Geometry check sheet. Reference: drawing and pictorial views, mm from the part's lowest x, y, z. Coordinates: 2 decimals unless noted, no trailing zeros. Write each loop counter-clockwise with the first axis right and the second up, starting at its lowest first coordinate (ties: lowest second). Pieces come first, ordered by that corner, then holes. Notation, with made-up numbers: (-14.5, 67.5) -> (14.5, 67.5) arc R20 ccw to (14.5, 81.5) -> close; hole circle Ø2 at (54.25, 17). An arc over 180 degrees is marked (long way). Use a Markdown table: item, result.
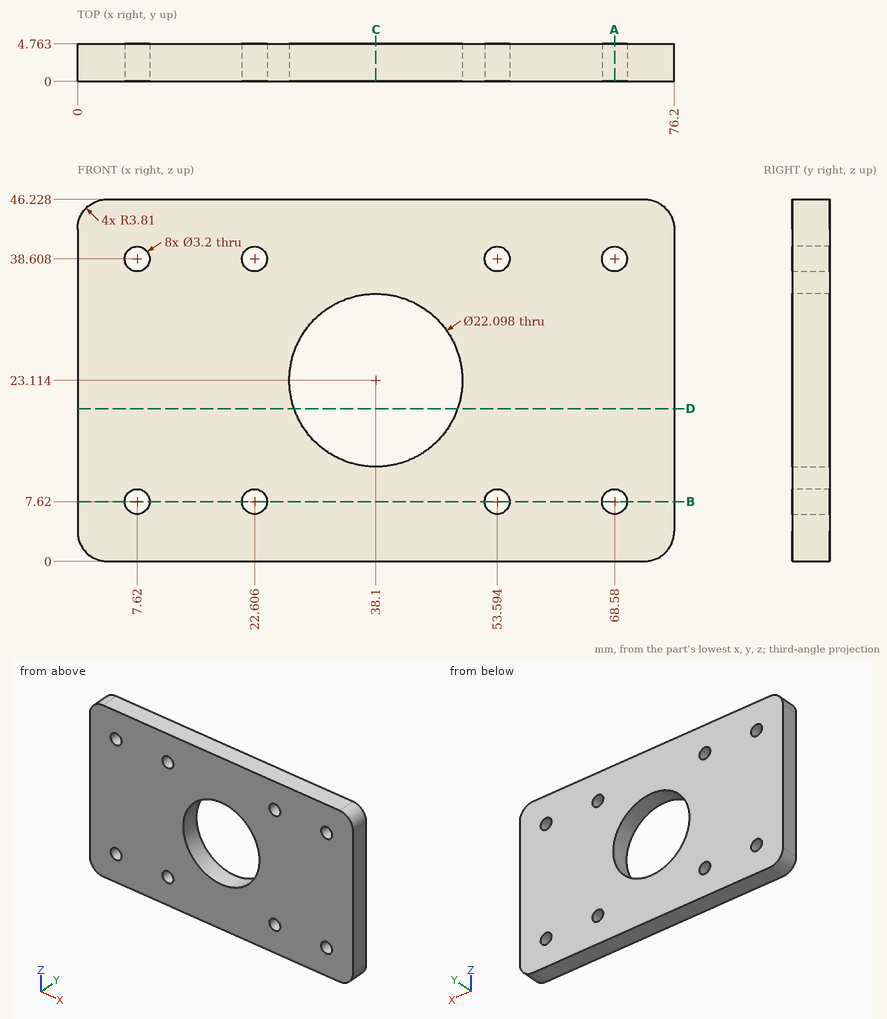
Item 1: Thickness scan on L1, parallel to X at y = 3.1, z = 7.62 (1 decimal); L2, parallel to Z at x = 68.5, y = 3.95 (1 decimal); L3, parallel to Z at x = 38.1, y = 1.3 (1 decimal). Record the ranges inside material, lowest first. Write a range as [from, to].
Answer block:
| item | result |
|---|---|
| L1 | x = [0, 6], [9.2, 21], [24.2, 52], [55.2, 67], [70.2, 76.2] |
| L2 | z = [0, 6], [9.2, 37], [40.2, 46.2] |
| L3 | z = [0, 12.1], [34.2, 46.2] |
Item 2: Section check B-B on z = 7.62. Record the boundary of the cut face in (x, y) (1 decimal), then the cut area to 3 significant figures.
Answer block:
| item | result |
|---|---|
| outline | (0, 0) -> (6, 0) -> (6, 4.8) -> (0, 4.8) -> close; (9.2, 0) -> (21, 0) -> (21, 4.8) -> (9.2, 4.8) -> close; (24.2, 0) -> (52, 0) -> (52, 4.8) -> (24.2, 4.8) -> close; (55.2, 0) -> (67, 0) -> (67, 4.8) -> (55.2, 4.8) -> close; (70.2, 0) -> (76.2, 0) -> (76.2, 4.8) -> (70.2, 4.8) -> close |
| area | 302 mm^2 |
Item 3: Section check A-A on x = 68.58. Record the boundary of the cut face in (y, z).
Answer block:
| item | result |
|---|---|
| outline | (0, 0) -> (4.76, 0) -> (4.76, 6.02) -> (0, 6.02) -> close; (0, 9.22) -> (4.76, 9.22) -> (4.76, 37.01) -> (0, 37.01) -> close; (0, 40.21) -> (4.76, 40.21) -> (4.76, 46.23) -> (0, 46.23) -> close |
Item 4: Section check D-D on z = 19.5. Record the boundary of the cut face in (x, y).
Answer block:
| item | result |
|---|---|
| outline | (0, 0) -> (27.66, 0) -> (27.66, 4.76) -> (0, 4.76) -> close; (48.54, 0) -> (76.2, 0) -> (76.2, 4.76) -> (48.54, 4.76) -> close |
Item 5: Section check C-C on x = 38.1. Record the boundary of the cut face in (y, z) (1 decimal), then the cut area to 3 significant figures.
Answer block:
| item | result |
|---|---|
| outline | (0, 0) -> (4.8, 0) -> (4.8, 12.1) -> (0, 12.1) -> close; (0, 34.2) -> (4.8, 34.2) -> (4.8, 46.2) -> (0, 46.2) -> close |
| area | 115 mm^2 |
